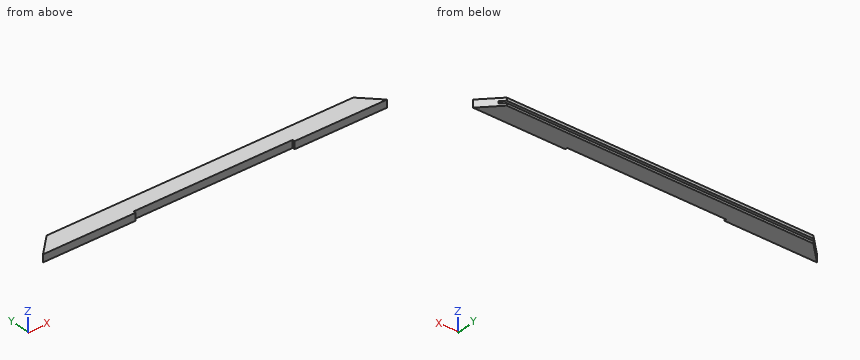
from build123d import *

# Parameters (mm, degrees)
F1_DEPTH = 20.6375
F2_W     = 12.7
F2_H     = 6.35
F3_DEPTH = 933.451
F4_W     = 431.8
F4_H     = 20.6375
F5_DEPTH = 6.35


with BuildPart() as f1:
    # F0 (on Top) → F1 (new body)
    with BuildSketch(Plane.XY):
        Polygon((50.8, 50.8), (0, 0), (933.45, 0), (882.65, 50.8), align=None)
    extrude(amount=F1_DEPTH)

    # F2 (on Right) → F3 (cut, through all)
    with BuildSketch(Plane.YZ):
        with Locations((44.45, 9.525)):
            Rectangle(F2_W, F2_H)
    extrude(amount=F3_DEPTH, mode=Mode.SUBTRACT)

    # F4 (on face) → F5 (cut)
    with BuildSketch(Plane.XZ):
        with Locations((466.725, 10.31875)):
            Rectangle(F4_W, F4_H)
    extrude(amount=-F5_DEPTH, mode=Mode.SUBTRACT)


solid = f1.part
Verification items for the finished model (mm, model axes). Round coordinates to 2 decimals unless told otherwise and drop trailing zeros. Loops run counter-clockwise (first coordinate to the right, second up) from the corner with the lowest first, then second, coordinate; pieces in that order, holes last. Notation, with made-up numbers: (62, 78.25) - (107, 78.25) arc R28 cw to (107, 96.25) - close; hole circle Ø7 at (53, 35.25). An arc over 180 degrees is marked (long way). Use one line per item in the form item = value.
1. Gauge pin test, flat ends, axial feed: pin 1 Ø2 at (x, z) = (168.5, 10) entering from +Y; pin 2 Ø1 at (y, z) = (15.5, 15) entering from +X; pin 3 Ø5 at (y, z) = (4.5, 9) entering from +X. Record the tip position at first contact, or that the pin passes through.
A:
pin_1 = 38.1
pin_2 = 918.45
pin_3 = 931.45
2. Section check C-C on y = 14. Record the cut outline in (x, z), and give its area (3 significant figures).
A:
outline = (14, 0) - (919.45, 0) - (919.45, 20.64) - (14, 20.64) - close
area = 18,700 mm²
3. Section check A-A on z = 9.5. Record the cut outline in (x, y) (3 decimals).
A:
outline = (0, 0) - (250.825, 0) - (250.825, 6.35) - (682.625, 6.35) - (682.625, 0) - (933.45, 0) - (895.35, 38.1) - (38.1, 38.1) - close
4. Scan lines: probe 1 along Z at (x, y) = (692.5, 43); probe 2 along Y at (x, z) = (717.5, 7.75); probe 3 along Y at (x, z) = (572, 18.5). Record each from-to range of solid material in increasing order.
A:
probe_1 = 0 to 6.35, 12.7 to 20.64
probe_2 = 0 to 38.1
probe_3 = 6.35 to 50.8
5. Section check B-B on x = 393. Record the cut outline in (y, z).
A:
outline = (6.35, 0) - (50.8, 0) - (50.8, 6.35) - (38.1, 6.35) - (38.1, 12.7) - (50.8, 12.7) - (50.8, 20.64) - (6.35, 20.64) - close
